from build123d import *

# Parameters (mm, degrees)
SKETCH_1_R          = 6
EXTRUDE_1_DEPTH     = 1.5
SKETCH_2_W          = 3.5
SKETCH_2_H          = 7
SKETCH_2_H_2        = 1.5
EXTRUDE_2_DEPTH     = 3
SKETCH_3_R          = 0.625
CUT_EXTRUDE_1_DEPTH = 4
FILLET_1_R          = 0.5
SKETCH_4_R          = 1.55
SKETCH_4_W          = 2.95
SKETCH_4_H          = 7
CUT_EXTRUDE_2_DEPTH = 4
SKETCH_5_R          = 0.75
CUT_EXTRUDE_3_DEPTH = 4
CUT_EXTRUDE_4_DEPTH = 4
FILLET_2_R          = 0.6
CUT_EXTRUDE_5_DEPTH = 4
FILLET_3_R          = 1
EXTRUDE_3_DEPTH     = 3
FILLET_4_R          = 0.8
CHAMFER_1_SIZE      = 2
FILLET_6_R          = 2


with BuildPart() as part:
    # 草图1 → 凸台-拉伸1 (new body, symmetric)
    with BuildSketch(Plane.XY):
        with BuildLine():
            Line((-5, 19), (6.237156693, 5.009778077))
            ThreePointArc((6.237156693, 5.009778077), (6.557579277, -4.582374279), (-2.56, -7.579340341))
            Line((-2.56, -7.579340341), (-25, 0))
            Line((-25, 0), (-25, 19))
            Line((-25, 19), (-5, 19))
        make_face()
        Circle(SKETCH_1_R, mode=Mode.SUBTRACT)
    extrude(amount=EXTRUDE_1_DEPTH, both=True)

    # 草图2 → 凸台-拉伸2 (add)
    with BuildSketch(Plane.XY.offset(1.5)):
        with Locations((-26.75, 9.5)):
            Rectangle(SKETCH_2_W, SKETCH_2_H)
        with Locations((-26.75, 2)):
            Rectangle(SKETCH_2_W, SKETCH_2_H_2)
        with Locations((-26.75, 17)):
            Rectangle(SKETCH_2_W, SKETCH_2_H_2)
    extrude(amount=-EXTRUDE_2_DEPTH)

    # 草图3 → 切除-拉伸1 (cut, through all)
    with BuildSketch(Plane.XY.offset(1.5)):
        with Locations((-25, 15.625)):
            Circle(SKETCH_3_R)
        with Locations((-25, 18.375)):
            Circle(SKETCH_3_R)
        with Locations((-25, 3.375)):
            Circle(SKETCH_3_R)
        with Locations((-25, 0.625)):
            Circle(SKETCH_3_R)
        with Locations((-25.625, 6)):
            Circle(SKETCH_3_R)
        with Locations((-25.625, 13)):
            Circle(SKETCH_3_R)
    extrude(amount=-CUT_EXTRUDE_1_DEPTH, mode=Mode.SUBTRACT)

    # 圆角1
    fillet_1_edges = [part.edges().sort_by_distance(p)[0] for p in [
        (-28.5, 6, 0),
        (-28.5, 13, 0),
        (-25, 19, 0),
    ]]
    fillet(fillet_1_edges, radius=FILLET_1_R)

    # 草图4 → 切除-拉伸2 (cut, through all)
    with BuildSketch(Plane(origin=(0, 0, -1.5), x_dir=(-1, 0, 0), z_dir=(0, 0, -1))):
        with Locations((17, 15.5)):
            Circle(SKETCH_4_R)
        with Locations((17, 3.5)):
            Circle(SKETCH_4_R)
        with Locations((8.5, 9.5)):
            Rectangle(SKETCH_4_W, SKETCH_4_H)
    extrude(amount=-CUT_EXTRUDE_2_DEPTH, mode=Mode.SUBTRACT)

    # 草图5 → 切除-拉伸3 (cut, through all)
    with BuildSketch(Plane(origin=(0, 0, -1.5), x_dir=(-1, 0, 0), z_dir=(0, 0, -1))):
        with Locations((7.025, 12.25)):
            Circle(SKETCH_5_R)
        with Locations((9.975, 12.25)):
            Circle(SKETCH_5_R)
        with Locations((7.025, 6.75)):
            Circle(SKETCH_5_R)
        with Locations((9.975, 6.75)):
            Circle(SKETCH_5_R)
    extrude(amount=-CUT_EXTRUDE_3_DEPTH, mode=Mode.SUBTRACT)

    # 草图6 → 切除-拉伸4 (cut, through all)
    with BuildSketch(Plane(origin=(0, 0, -1.5), x_dir=(-1, 0, 0), z_dir=(0, 0, -1))):
        with BuildLine():
            Line((12.475, 14), (12.475, 5))
            Line((12.475, 5), (13.782469891, 5))
            ThreePointArc((13.782469891, 5), (17, 7.05), (20.217530109, 5))
            Line((20.217530109, 5), (22.5, 5))
            Line((22.5, 5), (22.5, 14))
            Line((22.5, 14), (20.217530109, 14))
            ThreePointArc((20.217530109, 14), (17, 11.95), (13.782469891, 14))
            Line((13.782469891, 14), (12.475, 14))
        make_face()
    extrude(amount=-CUT_EXTRUDE_4_DEPTH, mode=Mode.SUBTRACT)

    # 圆角2
    fillet_2_edges = [part.edges().sort_by_distance(p)[0] for p in [
        (-12.475, 14, 0),
        (-13.782469891, 14, 0),
        (-20.217530109, 14, 0),
        (-22.5, 14, 0),
        (-22.5, 5, 0),
        (-20.217530109, 5, 0),
        (-13.782469891, 5, 0),
        (-12.475, 5, 0),
    ]]
    fillet(fillet_2_edges, radius=FILLET_2_R)

    # 草图7 → 切除-拉伸5 (cut, through all)
    with BuildSketch(Plane(origin=(0, 0, -1.5), x_dir=(-1, 0, 0), z_dir=(0, 0, -1))):
        with BuildLine():
            Line((7.193747285, 3.5), (13.305747104, 3.5))
            Line((13.305747104, 3.5), (14.604346249, -0.344736281))
            Line((14.604346249, -0.344736281), (7.516620657, -2.738688353))
            ThreePointArc((7.516620657, -2.738688353), (7.989307814, 0.413473892), (7.193747285, 3.5))
        make_face()
        with BuildLine():
            Line((4.525, 13.617995246), (0.012533825, 7.999990181))
            ThreePointArc((0.012533825, 7.999990181), (2.374697418, 7.639424859), (4.525, 6.597300584))
            Line((4.525, 6.597300584), (4.525, 13.617995246))
        make_face()
    extrude(amount=-CUT_EXTRUDE_5_DEPTH, mode=Mode.SUBTRACT)

    # 圆角3
    fillet_3_edges = [part.edges().sort_by_distance(p)[0] for p in [
        (-7.516620657, -2.738688353, 0),
        (-7.193747285, 3.5, 0),
        (-13.305747104, 3.5, 0),
        (-14.604346249, -0.344736281, 0),
        (-4.525, 13.617995246, 0),
        (-4.525, 6.597300584, 0),
        (-0.012533825, 7.999990181, 0),
    ]]
    fillet(fillet_3_edges, radius=FILLET_3_R)

    # 草图8 → 凸台-拉伸3 (add)
    with BuildSketch(Plane.XY.offset(1.5)):
        with BuildLine():
            Line((-25, 0), (-25, -8))
            Line((-25, -8), (0, -8))
            ThreePointArc((0, -8), (-1.297165617, -7.894134618), (-2.56, -7.579340341))
            Line((-2.56, -7.579340341), (-8.716260987, -5.5))
            Line((-8.716260987, -5.5), (-22.5, -5.5))
            Line((-22.5, -5.5), (-22.5, -0.844400662))
            Line((-22.5, -0.844400662), (-25, 0))
        make_face()
    extrude(amount=-EXTRUDE_3_DEPTH)

    # 圆角4
    fillet_4_edges = [part.edges().sort_by_distance(p)[0] for p in [
        (-22.5, -0.844400662, 0),
        (-22.5, -5.5, 0),
        (-8.716260987, -5.5, 0),
    ]]
    fillet(fillet_4_edges, radius=FILLET_4_R)

    # 倒角1
    chamfer_1_edges = [part.edges().sort_by_distance(p)[0] for p in [
        (-25, -8, 0),
    ]]
    chamfer(chamfer_1_edges, length=CHAMFER_1_SIZE)

    # 圆角6
    fillet_6_edges = [part.edges().sort_by_distance(p)[0] for p in [
        (-5, 19, 0),
    ]]
    fillet(fillet_6_edges, radius=FILLET_6_R)


solid = part.part
CAD build for the part. Positions are in the model's coordinates, mm. A direction names the side the tool comes from. Round coordinates to 2 decimals unless told otherwise and drop trailing zeros. Write each loop counter-clockwise with the first axis right and the second up, starting at its lowest first coordinate (ties: lowest second). Pieces come first, ordered by that corner, then holes. Notation, with made-up numbers: M -2,77 L 46,77 A16 ccw 46,81 Z; hole C 6.25,16 d5. An arc over 180 degrees is marked long. Put each result on its own line as item: value. Start each with the question number.
1) 3-axis set-ups, long thin cutter, end or side, ignore diameter. For faces 4 (the flat face through (-13.905, 1.727, -0.021)), 5 (the cylindrical face through (-24.375, 3.361, 0.021)): which of +Z, -Z, +X, -X, +Y, -Y reach the whole face in a straight line?
2) Drill centre lines: probe 1 along Y at (x, z) = (-9, -1); probe 2 along Y at (x, z) = (-10.5, 0.2); probe 3 along X at (y, z) = (12.75, 0.75) (3 decimals). Where is each one in solid material? Low to high. Write a range as [from, to].
3) Saw through at A-A, the plane y = 4.5. Write the cut outline in (x, z).
4) Saw through at D-D, the plane z = 0.75. Count the separate pieces of the cut face and the enclosed holes in it, and give its area (3 significant figures).
5) Saw through at C-C, the plane x = 2. Write the cut outline in (y, z), and give its area (3 significant figures).
6) Pull direction Y, two halves, no side cores. Call faces 1 (the flat face through (-25, 5, 0)), 2 (the flat face through (-12, -8, 0)), 3 (the flat face through (-15, 6, 1.5)): pulls with the +Y half, pulls with the -Y half, needs draft (parallel to the pull), parting line crosses it, or undercut.
7) Pin check, flat tips, straight feed: pin 1 Ø0.8 at (y, z) = (-3, 0) entering from +X; pin 2 Ø1.5 at (y, z) = (11, -0.5) entering from +X; pin 3 Ø1.5 at (y, z) = (-3.5, 0.5) entering from -X; pin 4 Ø1.5 at (x, y) = (-8, 11.5) entering from +Z. Stop position of each tip, or through.
8) Saw through at B-B, the plane x = -25.5. Write the cut outline in (y, z).
Resolved:
1. face 4: +Z, -Z
1. face 5: +Z, -Z, -X
2. probe 1: [-8, -2.21], [3.5, 6], [13, 19]
2. probe 2: [-8, -1.73], [3.5, 6.21], [7.29, 11.71], [12.79, 19]
2. probe 3: [-28.433, -26.198], [-25.052, -22.5], [-19.245, -14.755], [-12.475, -10.534], [-6.466, 0.02]
3. outline: M -25,-1.5 L -18.18,-1.5 L -18.18,1.5 L -25,1.5 Z; M -15.82,-1.5 L -3.97,-1.5 L -3.97,1.5 L -15.82,1.5 Z; M 3.97,-1.5 L 6.61,-1.5 L 6.61,1.5 L 3.97,1.5 Z
4. separate pieces: 1
4. enclosed holes: 8
4. area: 506 mm²
5. outline: M -7.75,-1.5 L -5.66,-1.5 L -5.66,1.5 L -7.75,1.5 Z; M 5.66,-1.5 L 10.29,-1.5 L 10.29,1.5 L 5.66,1.5 Z
5. area: 20.2 mm²
6. face 1: undercut
6. face 2: pulls with the -Y half
6. face 3: needs draft
7. pin 1: x = 7.57
7. pin 2: x = 2.03
7. pin 3: x = -25
7. pin 4: through
8. outline: M 1.25,-1.5 L 2.75,-1.5 L 2.75,1.5 L 1.25,1.5 Z; M 6.61,-1.5 L 12.39,-1.5 L 12.39,1.5 L 6.61,1.5 Z; M 16.25,-1.5 L 17.75,-1.5 L 17.75,1.5 L 16.25,1.5 Z
